```python
from build123d import *

# Parameters (mm, degrees)
F0_W     = 16.891
F0_H     = 26.0096
F1_DEPTH = 44.704
F2_R     = 2.5019
F2_R_2   = 4.0005
F3_DEPTH = 3.9878
F4_R     = 1.27


with BuildPart() as f1:
    # F0 (on Top) → F1 (new body)
    with BuildSketch(Plane.XY):
        Rectangle(F0_W, F0_H)
    extrude(amount=F1_DEPTH)

    # F2 (on Top) → F3 (join)
    with BuildSketch(Plane.XY):
        with Locations((0, 7.796854)):
            Circle(F2_R)
        with Locations((0, -5.207946)):
            Circle(F2_R_2)
    extrude(amount=-F3_DEPTH)

    # F4
    f4_edges = [f1.edges().sort_by_distance(p)[0] for p in [
        (0, -13.0048, 0),
        (-8.4455, 0, 0),
        (0, 13.0048, 0),
        (8.4455, 0, 0),
        (-8.4455, -13.0048, 22.352),
        (-8.4455, 13.0048, 22.352),
        (8.4455, -13.0048, 22.352),
        (0, -13.0048, 44.704),
        (-8.4455, 0, 44.704),
        (8.4455, 13.0048, 22.352),
        (8.4455, 0, 44.704),
        (0, 13.0048, 44.704),
    ]]
    fillet(f4_edges, radius=F4_R)


solid = f1.part
```
The model under review builds one solid part; all positions refer to its coordinate system, in mm. Give positions to 0.01 mm unless a question says otherwise; leave off trailing zeros. Write each loop counter-clockwise with the first axis right and the second up, starting at its lowest first coordinate (ties: lowest second). Pieces come first, ordered by that corner, then holes. Notation, with made-up numbers: (53.25, 46) -> (61.25, 46) arc R13 cw to (61.25, 67) -> close; hole circle Ø4 at (30, 49). An arc over 180 degrees is marked (long way). Answer in a Markdown table with one row per item.
1) Add section D-D on y = -7.5. State the section outline as (x, z) points.
Worked answers:
| item | result |
|---|---|
| outline | (-8.45, 1.27) arc R1.27 ccw to (-7.18, 0) -> (-3.28, 0) -> (-3.28, -3.99) -> (3.28, -3.99) -> (3.28, 0) -> (7.18, 0) arc R1.27 ccw to (8.45, 1.27) -> (8.45, 43.43) arc R1.27 ccw to (7.18, 44.7) -> (-7.18, 44.7) arc R1.27 ccw to (-8.45, 43.43) -> close |
2) For L1, parallel to Z at x = 1.5, y = 10; L2, parallel to Y at x = 5.75, z = 43.5; L3, parallel to Z at x = 7.75, y = 2.75, list the stretches that pass through material, from the lowest coordinate up. Write a range as [from, to].
Worked answers:
| item | result |
|---|---|
| L1 | [0, 44.7] |
| L2 | [-13, 13] |
| L3 | [0.14, 44.57] |
3) Mouldability with a two-part tool opening along Y and no side actions: class faces 1 (the cylindrical face through (8.064, 12.643, 22.647)), 2 (the flat face through (-8.446, 0, 22)), 3 (the cylindrical face through (-0.542, 5.354, -1.966)) as +Y half, -Y half, draft (parallel to the pull), parting line (faces both ways), or undercut.
Worked answers:
| item | result |
|---|---|
| face 1 | +Y half |
| face 2 | draft |
| face 3 | undercut |
4) Add section C-C on x = 5. State the section outline as (y, z) points.
Worked answers:
| item | result |
|---|---|
| outline | (-13, 1.27) arc R1.27 ccw to (-11.73, 0) -> (11.73, 0) arc R1.27 ccw to (13, 1.27) -> (13, 43.43) arc R1.27 ccw to (11.73, 44.7) -> (-11.73, 44.7) arc R1.27 ccw to (-13, 43.43) -> close |
5) Add section A-A on x = 0. State the section outline as (y, z) points, plus the area to 3 significant figures.
Worked answers:
| item | result |
|---|---|
| outline | (-13, 1.27) arc R1.27 ccw to (-11.73, 0) -> (-9.21, 0) -> (-9.21, -3.99) -> (-1.21, -3.99) -> (-1.21, 0) -> (5.29, 0) -> (5.29, -3.99) -> (10.3, -3.99) -> (10.3, 0) -> (11.73, 0) arc R1.27 ccw to (13, 1.27) -> (13, 43.43) arc R1.27 ccw to (11.73, 44.7) -> (-11.73, 44.7) arc R1.27 ccw to (-13, 43.43) -> close |
| area | 1,210 mm² |
6) Add section B-B on y = 2. State the section outline as (x, z) points.
Worked answers:
| item | result |
|---|---|
| outline | (-8.45, 1.27) arc R1.27 ccw to (-7.18, 0) -> (7.18, 0) arc R1.27 ccw to (8.45, 1.27) -> (8.45, 43.43) arc R1.27 ccw to (7.18, 44.7) -> (-7.18, 44.7) arc R1.27 ccw to (-8.45, 43.43) -> close |
